from build123d import *

# Parameters (mm, degrees)
BOSS_EXTRUDE4_DEPTH = 16.5
CUT_EXTRUDE2_DEPTH  = 1.5
CUT_EXTRUDE4_DEPTH  = 17.5
SKETCH6_W           = 12
SKETCH6_H           = 2
CUT_EXTRUDE5_DEPTH  = 17.5
BOSS_EXTRUDE5_DEPTH = 2
SKETCH10_R          = 2.38125
CUT_EXTRUDE6_DEPTH  = 13.606601718
CUT_EXTRUDE7_DEPTH  = 17.5
SKETCH12_R          = 2.38125
CUT_EXTRUDE8_DEPTH  = 6.35
SKETCH13_R          = 4.5
CUT_EXTRUDE13_DEPTH = 20
SKETCH14_W          = 6.5
SKETCH14_H          = 9
CUT_EXTRUDE14_DEPTH = 6


with BuildPart() as part:
    # Sketch1 → Boss-Extrude4 (new body)
    with BuildSketch(Plane(origin=(0, 0, 0), x_dir=(0, 0, -1), z_dir=(1, 0, 0))):
        Polygon((0, 0), (0, 37.1), (-10.606601718, 47.706601718), (12, 47.706601718), (12, 0), align=None)
    extrude(amount=BOSS_EXTRUDE4_DEPTH)

    # Sketch4 → Cut-Extrude2 (cut)
    with BuildSketch(Plane.ZY):
        Polygon((0, 37.1), (0, 47.706601718), (10.606601718, 47.706601718), align=None)
    extrude(amount=-CUT_EXTRUDE2_DEPTH, mode=Mode.SUBTRACT)

    # Sketch5 → Cut-Extrude4 (cut, through all)
    with BuildSketch(Plane(origin=(16.5, 0, 0), x_dir=(0, 0, -1), z_dir=(1, 0, 0))):
        Polygon((-3.566952421, 40.666952421), (-2.859845639, 39.959845639), (-1.799185468, 41.020505811), (0, 39.221320344), (0, 42.756854249), (-2.683068944, 45.439923194), (-4.450835897, 43.672156241), (-3.036622335, 42.257942678), (-4.097282506, 41.197282506), align=None)
    extrude(amount=-CUT_EXTRUDE4_DEPTH, mode=Mode.SUBTRACT)

    # Sketch6 → Cut-Extrude5 (cut, through all)
    with BuildSketch(Plane(origin=(16.5, 0, 0), x_dir=(0, 0, -1), z_dir=(1, 0, 0))):
        with Locations((6, 1)):
            Rectangle(SKETCH6_W, SKETCH6_H)
    extrude(amount=-CUT_EXTRUDE5_DEPTH, mode=Mode.SUBTRACT)

    # Sketch9 → Boss-Extrude5 (add)
    with BuildSketch(Plane.XY):
        with BuildLine():
            Line((16.5, 29), (16.5, 25))
            Line((16.5, 25), (20.518219338, 25))
            ThreePointArc((20.518219338, 25), (24.518219338, 29), (20.518219338, 33))
            Line((20.518219338, 33), (16.5, 33))
            Line((16.5, 33), (16.5, 29))
        make_face()
    extrude(amount=-BOSS_EXTRUDE5_DEPTH)

    # Sketch10 → Cut-Extrude6 (cut, through all)
    with BuildSketch(Plane(origin=(0, 0, -2), x_dir=(-1, 0, 0), z_dir=(0, 0, -1))):
        with Locations((-20.518219338, 29)):
            Circle(SKETCH10_R)
    extrude(amount=-CUT_EXTRUDE6_DEPTH, mode=Mode.SUBTRACT)

    # Sketch11 → Cut-Extrude7 (cut, through all)
    with BuildSketch(Plane(origin=(16.5, 0, 0), x_dir=(0, 0, -1), z_dir=(1, 0, 0))):
        Polygon((0, 37.1), (-10.606601718, 47.706601718), (12, 47.706601718), (12, 37.1), align=None)
    extrude(amount=-CUT_EXTRUDE7_DEPTH, mode=Mode.SUBTRACT)

    # Sketch12 → Cut-Extrude8 (cut)
    with BuildSketch(Plane.XZ.offset(-2)):
        with Locations((8.25, -6)):
            Circle(SKETCH12_R)
    extrude(amount=-CUT_EXTRUDE8_DEPTH, mode=Mode.SUBTRACT)

    # Sketch13 → Cut-Extrude13 (cut)
    with BuildSketch(Plane(origin=(0, 37.1, 0), x_dir=(1, 0, 0), z_dir=(0, 1, 0))):
        with Locations((6, 5)):
            Circle(SKETCH13_R)
    extrude(amount=-CUT_EXTRUDE13_DEPTH, mode=Mode.SUBTRACT)

    # Sketch14 → Cut-Extrude14 (cut)
    with BuildSketch(Plane.XY):
        with Locations((6.25, 25.5)):
            Rectangle(SKETCH14_W, SKETCH14_H)
    extrude(amount=-CUT_EXTRUDE14_DEPTH, mode=Mode.SUBTRACT)


solid = part.part
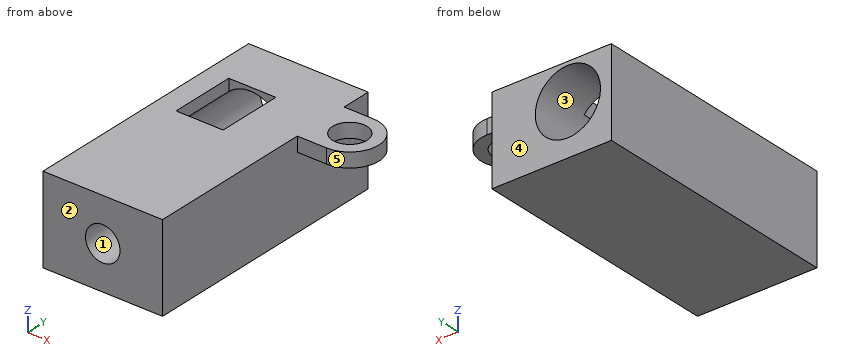
Geometry check sheet. Reference: the model listing, model coordinates, mm. Face numbers are marked on the shaded views. A direction names the side the tool comes from. Coordinates: 2 decimals unless noted, no trailing zeros. Order: outer loops, then holes, each group sorted by start corner. A loop starts at its lowest first (then second) coordinate and runs counter-clockwise, first axis right, second up. Notation, with made-up numbers: (79, 74) -> (124, 74) arc R31 ccw to (124, 111) -> close; hole circle Ø3 at (50.25, -2). An arc over 180 degrees is marked (long way). Use a Markdown table: item, result. Add a question column.
1. Cross-section at D-D (y = 14). Enter the section's corners in (x, z).
2. Cross-section at A-A (y = 30.5). Enter the section's corners in (x, z).
3. Material ranges on L1, parallel to X at y = 32, z = -5; L2, parallel to Z at x = 8.25, y = 6.75; L3, parallel to X at y = 32.5, z = -11.5, recorded low to high.
4. Mould release check, pull along X, two halves, no side actions. Record for the marked faces 3, 4 and 5: pulls with the +X half, pulls with the -X half, needs draft (parallel to the pull), parting line crosses it, or undercut.
5. Go/stop test with flat-tipped pins: pin 1 Ø2 at (x, z) = (19, -1.5) entering from -Y; pin 2 Ø4 at (x, y) = (20.52, 29) entering from +Z; pin 3 Ø1.6 at (x, z) = (19.5, -1.5) entering from +Y; pin 4 Ø4.5 at (x, z) = (6.5, -3) entering from +Y. Record where each tip stops, or that it passes through.
6. Set-up check for the marked faces 1 and 2: record each of +Z, -Z, +X, -X, +Y, -Y from which the full face is reachable in a straight line by a thin tool's end or side.
7. Cross-section at C-C (z = -6). Enter the section's corners in (x, y).
8. Cross-section at B-B (x = 5.5). Enter the section's corners in (y, z), and give its area (3 significant figures).
Filled sheet:
| question | item | result |
|---|---|---|
| 1 | outline | (0, -12) -> (16.5, -12) -> (16.5, 0) -> (0, 0) -> close |
| 2 | outline | (0, -12) -> (16.5, -12) -> (16.5, -2) -> (18.67, -2) -> (18.67, 0) -> (0, 0) -> close; (22.37, -2) -> (24.23, -2) -> (24.23, 0) -> (22.37, 0) -> close; hole circle Ø9 at (6, -5) |
| 3 | L1 | 0 to 1.5, 10.5 to 16.5 |
| 3 | L2 | -12 to -8.38, -3.62 to 0 |
| 3 | L3 | 0 to 16.5 |
| 4 | face 3 | undercut |
| 4 | face 4 | needs draft |
| 4 | face 5 | pulls with the +X half |
| 5 | pin 1 | y = 25 |
| 5 | pin 2 | through |
| 5 | pin 3 | y = 33 |
| 5 | pin 4 | y = 17.1 |
| 6 | face 1 | -Y |
| 6 | face 2 | +Z, -Z, +X, -X, -Y |
| 7 | outline | (0, 2) -> (5.87, 2) -> (5.87, 8.35) -> (10.63, 8.35) -> (10.63, 2) -> (16.5, 2) -> (16.5, 37.1) -> (10.39, 37.1) -> (10.39, 17.1) -> (1.61, 17.1) -> (1.61, 37.1) -> (0, 37.1) -> close |
| 8 | outline | (2, -12) -> (37.1, -12) -> (37.1, -9.47) -> (17.1, -9.47) -> (17.1, -0.53) -> (21, -0.53) -> (21, 0) -> (2, 0) -> close; (30, -0.53) -> (37.1, -0.53) -> (37.1, 0) -> (30, 0) -> close |
| 8 | area | 238 mm2 |
